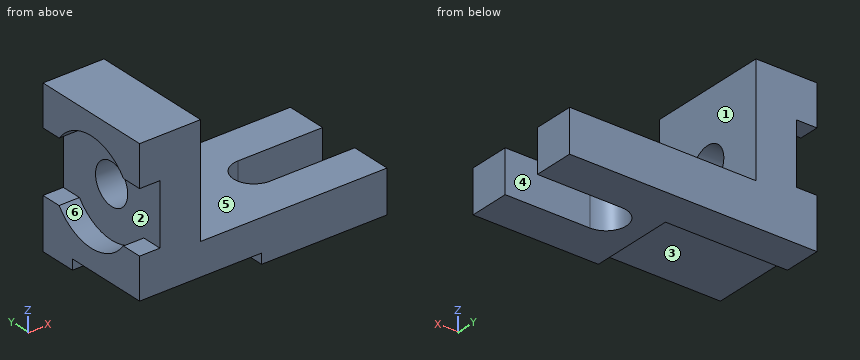
Autodesk Fusion 360 part; units mm, degrees
sketch "Sketch1" plane through (0, 0, 0) normal (0, 0, 1) x (1, 0, 0)
  line L0 (73, 36) -> (-73, 36)
  line L1 (-73, 36) -> (-73, -36)
  line L2 (-73, -36) -> (73, -36)
  line L3 (73, -36) -> (73, 36)
  line L4 (73, 36) -> (-73, -36) construction
  line L5 (-73, 36) -> (73, -36) construction
  line L6 (-73, -36) -> (-1, -36)
  line L7 (-1, -36) -> (-1, 14)
  line L8 (-1, 14) -> (-73, 14)
  line L9 (-73, 14) -> (-73, -36)
  line L10 (23, 12) -> (73, 12)
  line L11 (23, -12) -> (73, -12)
  arc A0 (24.2094, 11.9389) -> (24.2094, -11.9389) centre (23, 0) ccw
  dimension "d1" = 146
  dimension "d2" = 72
  dimension "d3" = 72
  dimension "d4" = 50
  dimension "d5" = 24
  dimension "d6" = 50
extrude "Extrude1" add sketch "Sketch1" along normal blind 25 contours L0 L1 L2 L3 L7 L8 L10 L11 A0 | L1 L2 L6 L7 L8 L9
extrude "Extrude2" cut sketch "Sketch1" along normal blind 6 contours L1 L2 L6 L7 L8 L9
sketch "Sketch2" plane through (0, 0, 25) normal (0, 0, 1) x (-1, 0, 0)
  arc A0 (-23, -12) -> (-23, 12) centre (-23, 0) ccw
  line L0 (-23, -12) -> (-73, -12)
  line L1 (-73, -12) -> (-73, -36)
  line L2 (-73, -36) -> (73, -36)
  line L3 (73, -36) -> (73, 36)
  line L4 (73, 36) -> (-73, 36)
  line L5 (-73, 36) -> (-73, 12)
  line L6 (-73, 12) -> (-23, 12)
  line L7 (73, -36) -> (37, -36)
  line L8 (37, -36) -> (37, 36)
  line L9 (37, 36) -> (73, 36)
  line L10 (73, 36) -> (73, -36)
  dimension "d11" = 36
extrude "Extrude3" add sketch "Sketch2" along normal blind 65 contours L2 L3 L4 L7 L8 L9 L10
sketch "Sketch3" plane through (-73, 0, 0) normal (-1, 0, 0) x (0, -1, 0)
  line L0 (-14, 0) -> (-14, 6)
  line L1 (-14, 6) -> (36, 6)
  line L2 (36, 6) -> (36, 90)
  line L3 (36, 90) -> (-36, 90)
  line L4 (-36, 90) -> (-36, 0)
  line L5 (-36, 0) -> (-14, 0)
  circle A0 centre (0, 48) radius 12
  circle A1 centre (0, 48) radius 30
  line L6 (-36, 90) -> (36, 90)
  line L7 (36, 90) -> (36, 66)
  line L8 (36, 66) -> (-36, 66)
  line L9 (-36, 66) -> (-36, 90)
  line L10 (36, 6) -> (-36, 6)
  line L11 (-36, 6) -> (-36, 30)
  line L12 (-36, 30) -> (36, 30)
  line L13 (36, 30) -> (36, 6)
  dimension "d14" = 24
  dimension "d15" = 60
  dimension "d16" = 48
  dimension "d17" = 24
  dimension "d18" = 24
extrude "Extrude4" cut sketch "Sketch3" against normal through all contours A0
extrude "Extrude5" cut sketch "Sketch3" against normal blind 12 contours L2 A1 L8 L12 | L4 A1 L8 L12 | A1 L8 L12 | A1 L12 | A1 L8
Model file for the job. Use its own axes, mm. Face numbers are marked on the shaded views. A direction names the side the tool comes from. Round coordinates to 2 decimals unless told otherwise and drop trailing zeros. Order: outer loops, then holes, each group sorted by start corner. A loop starts at its lowest first (then second) coordinate and runs counter-clockwise, first axis right, second up.
(1) Pull direction Z, two halves, no side cores. Call the marked faces 4, 5 and 6: released by +Z, released by -Z, zero draft, split by the parting line, or undercut.
(2) Drill centre lines: line 1 (Z direction, x = -42.25, y = 0); line 2 (Z direction, x = -63, y = 28); line 3 (X direction, y = 32.5, z = 64). Where is each one in solid material? Low to high.
(3) 3-axis set-ups, long thin cutter, end or side, ignore diameter. For the marked faces 1, 2 and 3: which of +Z, -Z, +X, -X, +Y, -Y reach the whole face in a straight line?
(4) Band-saw the part on D-D (x = -45). List the corners of the cut face in (y, z), then the cut area to 3 significant figures.
(5) Band-saw the part on C-C (y = 0). List the corners of the cut face in (x, z).
(6) Pin check, flat tips, straight feed: pin 1 (5 mm diameter, centred on y = -6, z = 1.5, fed in from -X); pin 2 (3.5 mm diameter, centred on x = -65.5, y = -29.5, fed in from -Z). Stop position of each tip, or through.
(7) Band-saw the part on B-B (z = 48). List the corners of the cut face in (x, y).
(8) Band-saw the part on A-A (x = 26). List the corners of the cut face in (y, z).
Verdict:
1. face 4: zero draft
1. face 5: released by +Z
1. face 6: undercut
2. line 1: z = 6 to 36, 60 to 90
2. line 2: z = 0 to 30, 66 to 90
2. line 3: x = -61 to -37
3. face 1: +Z, +X, +Y, -Y
3. face 2: -X
3. face 3: -Z, -X, -Y
4. outline: (-36, 6) - (14, 6) - (14, 0) - (36, 0) - (36, 90) - (-36, 90) - close; hole circle Ø24 at (0, 48)
4. area: 5,730 mm2
5. outline: (-73, 6) - (-1, 6) - (-1, 0) - (11, 0) - (11, 25) - (-37, 25) - (-37, 36) - (-61, 36) - (-61, 18) - (-73, 18) - close; (-73, 78) - (-61, 78) - (-61, 60) - (-37, 60) - (-37, 90) - (-73, 90) - close
6. pin 1: stops at x = -1
6. pin 2: stops at z = 6
7. outline: (-61, -36) - (-37, -36) - (-37, -12) - (-61, -12) - close; (-61, 12) - (-37, 12) - (-37, 36) - (-61, 36) - close
8. outline: (-36, 0) - (-12, 0) - (-12, 25) - (-36, 25) - close; (12, 0) - (36, 0) - (36, 25) - (12, 25) - close
